Can you work these out from the model? Positions are in its coordinate system, mm. Face numbers are marked on the shaded views. A direction names the side the tool comes from. Give positions to 0.01 mm unless a question says otherwise; leave off trailing zeros. Order: outer loops, then holes, each group sorted by start corner. A loop starts at its lowest first (then second) coordinate and runs counter-clockwise, first axis right, second up. Notation, with made-up numbers: M -22.75,-39.5 L 32.25,-39.5 A29 ccw 32.25,-0.5 Z; hole C 2,48.25 d2. An arc over 180 degrees is marked long. Answer as a JSON object with one key per item and string values.
```python
from build123d import *

# Parameters (mm, degrees)
SKETCH2_R           = 12
BOSS_EXTRUDE1_DEPTH = 12
SKETCH4_W           = 15.195212274
SKETCH4_H           = 7.463727614
SKETCH4_W_2         = 12.852338134
SKETCH4_H_2         = 4.920035692
BOSS_EXTRUDE2_DEPTH = 2
SKETCH5_W           = 11.647431434
SKETCH5_H           = 1.606542266
BOSS_EXTRUDE3_DEPTH = 2
SKETCH6_W           = 12.852338134
SKETCH6_H           = 4.920035692
SKETCH6_W_2         = 11.647431434
SKETCH6_H_2         = 1.606542266
CUT_EXTRUDE1_DEPTH  = 2


with BuildPart() as part:
    # Sketch2 → Boss-Extrude1 (new body)
    with BuildSketch(Plane.XY):
        Circle(SKETCH2_R)
    extrude(amount=BOSS_EXTRUDE1_DEPTH)

    # Sketch4 → Boss-Extrude2 (add)
    with BuildSketch(Plane.XY.offset(12)):
        Rectangle(SKETCH4_W, SKETCH4_H)
        Rectangle(SKETCH4_W_2, SKETCH4_H_2, mode=Mode.SUBTRACT)
    extrude(amount=BOSS_EXTRUDE2_DEPTH)

    # Sketch5 → Boss-Extrude3 (add)
    with BuildSketch(Plane.XY.offset(12)):
        with Locations((0, 1.020823732)):
            Rectangle(SKETCH5_W, SKETCH5_H)
    extrude(amount=BOSS_EXTRUDE3_DEPTH)

    # Sketch6 → Cut-Extrude1 (cut)
    with BuildSketch(Plane.XY.offset(12)):
        Rectangle(SKETCH6_W, SKETCH6_H)
        with Locations((0, 1.020823732)):
            Rectangle(SKETCH6_W_2, SKETCH6_H_2, mode=Mode.SUBTRACT)
    extrude(amount=-CUT_EXTRUDE1_DEPTH, mode=Mode.SUBTRACT)


solid = part.part
```
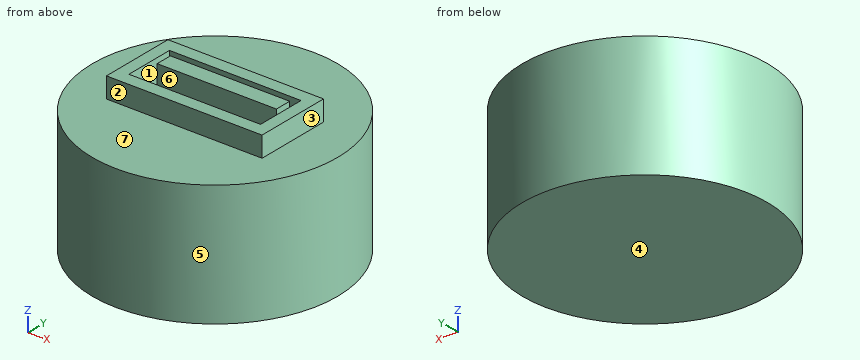
1) I want a section at C-C on z = 7.5. Write out the boundary of the cut face in (x, y).
Results found:
{"outline": "C 0,0 d24"}
2) I need wall thicknesses on L1, parallel to Y at x = -2, z = 13; L2, parallel to Z at x = -9.25, y = 5.5; L3, parallel to X at y = -2, z = 10.5. Which ranges of each line are inside material? Lowest first, please.
Results found:
{"L1": "y = -3.73 to -2.46, 0.22 to 1.82, 2.46 to 3.73", "L2": "z = 0 to 12", "L3": "x = -11.83 to -6.43, 6.43 to 11.83"}
3) I want a section at A-A on z = 13. Write out the boundary of the cut face in (x, y).
Results found:
{"outline": "M -7.6,-3.73 L 7.6,-3.73 L 7.6,3.73 L -7.6,3.73 Z; M -5.82,0.22 L 5.82,0.22 L 5.82,1.82 L -5.82,1.82 Z; hole M -6.43,-2.46 L 6.43,-2.46 L 6.43,2.46 L -6.43,2.46 Z"}
4) I want a section at B-B on x = 0. Write out the boundary of the cut face in (y, z).
Results found:
{"outline": "M -12,0 L 12,0 L 12,12 L 3.73,12 L 3.73,14 L 2.46,14 L 2.46,10 L 1.82,10 L 1.82,14 L 0.22,14 L 0.22,10 L -2.46,10 L -2.46,14 L -3.73,14 L -3.73,12 L -12,12 Z"}
5) Thinking about a two-plate mould opening in X: for the marked faces 5, 6 and 7, which applies, pulls with the +X half, pulls with the -X half, needs draft (parallel to the pull), parting line crosses it, or undercut?
Results found:
{"face 5": "parting line crosses it", "face 6": "undercut", "face 7": "needs draft"}
6) For the marked faces 1, 2, 3 and 4, which set-ups out of +Z, -Z, +X, -X, +Y, -Y let a thin tool reach every point of the face, with its end or its side?
Results found:
{"face 1": "+Z", "face 2": "+Z, +X, -X, -Y", "face 3": "+Z, +X, +Y, -Y", "face 4": "-Z, +X, -X, +Y, -Y"}
7) I'm going to push flat-ended pins straight in: pin 1 Ø5 at (x, z) = (-7, 12.5) entering from -Y; pin 2 Ø6 at (y, z) = (7.5, 1.5) entering from +X; pin 3 Ø3 at (x, y) = (7.5, -8) entering from +Z. Where does each tip first touch, or does it pass through?
Results found:
{"pin 1": "stops at y = -11.1", "pin 2": "stops at x = 11.12", "pin 3": "stops at z = 12"}
8) I want a section at D-D on y = -2. Write out the boundary of the cut face in (x, z), and give its area (3 significant figures).
Results found:
{"outline": "M -11.83,0 L 11.83,0 L 11.83,12 L 7.6,12 L 7.6,14 L 6.43,14 L 6.43,10 L -6.43,10 L -6.43,14 L -7.6,14 L -7.6,12 L -11.83,12 Z", "area": "263 mm²"}
